Geometry: see drawing. Coordinates: mm, zero at the bounding-box minimum. Give positions to 0.01 mm unless a question says otherwise; leave off trailing zeros. Loops run counter-clockwise (first coordinate to the right, second up) from the corner with the lowest first, then second, coordinate; pieces in that order, holes last. Notation, with made-up numbers: M 29.25,72 L 53.25,72 A24 ccw 53.25,103 Z; hole C -4,84 d6. An arc over 180 degrees is marked long. Answer in a Markdown table with one row per item.
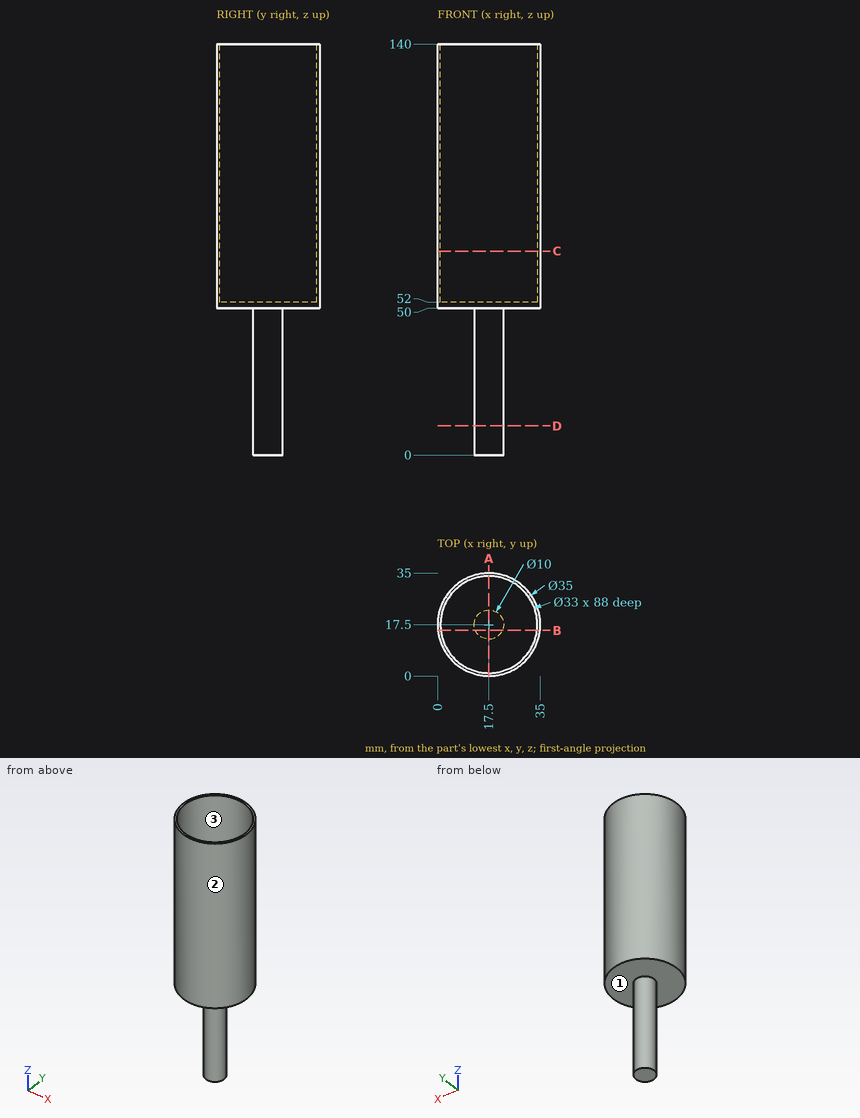
1) Pull-direction query (X, two-part tool) for the marked faces 1, 2 and 3; classes: released by +X, released by -X, zero draft, split by the parting line, or undercut.
Reply:
| item | result |
|---|---|
| face 1 | zero draft |
| face 2 | split by the parting line |
| face 3 | undercut |
2) Section C-C, the plane z = 69.5. Return loops of the section in (x, y).
Reply:
| item | result |
|---|---|
| outline | C 17.5,17.5 d35; hole C 17.5,17.5 d33 |
3) Section B-B, the plane y = 15.5. Return loops of the section in (x, z), then the cut area to 3 significant figures.
Reply:
| item | result |
|---|---|
| outline | M 0.11,50 L 12.92,50 L 12.92,0 L 22.08,0 L 22.08,50 L 34.89,50 L 34.89,140 L 33.88,140 L 33.88,52 L 1.12,52 L 1.12,140 L 0.11,140 Z |
| area | 705 mm² |
4) Material intervals for L1, parallel to Y at x = 17.5, z = 95.5; L2, parallel to X at y = 17, z = 113; L3, parallel to Z at x = 19.5, y = 21.5, sorted ascending.
Reply:
| item | result |
|---|---|
| L1 | y = 0 to 1, 34 to 35 |
| L2 | x = 0.01 to 1.01, 33.99 to 34.99 |
| L3 | z = 0 to 52 |
5) Pin query (flat end, axial travel): pin 1 Ø6 at (y, z) = (8.5, 64) entering from +X; pin 2 Ø6 at (x, y) = (30, 29) entering from -Z; pin 3 Ø6 at (y, z) = (22, 76) entering from +X. Return the tip coordinate at first contact, or that it passes through.
Reply:
| item | result |
|---|---|
| pin 1 | stops at x = 33.94 |
| pin 2 | stops at z = 50 |
| pin 3 | stops at x = 34.94 |
6) Section D-D, the plane z = 10. Return loops of the section in (x, y), then the cut area to 3 significant figures.
Reply:
| item | result |
|---|---|
| outline | C 17.5,17.5 d10 |
| area | 78.5 mm² |
7) Section A-A, the plane x = 17.5. Return loops of the section in (y, z).
Reply:
| item | result |
|---|---|
| outline | M 0,50 L 12.5,50 L 12.5,0 L 22.5,0 L 22.5,50 L 35,50 L 35,140 L 34,140 L 34,52 L 1,52 L 1,140 L 0,140 Z |
